from build123d import *

# Parameters (mm, degrees)
SKETCH_W            = 50
SKETCH_H            = 50
PAD_DEPTH           = 4
SKETCH001_W         = 50
SKETCH001_H         = 4
PAD001_DEPTH        = 43
SKETCH002_R         = 11.75
POCKET_DEPTH        = 4.001
HOLE_D              = 4.4
HOLE_CSINK_D        = 8
HOLE_CSINK_ANGLE    = 90
HOLE001_D           = 3.3
HOLE001_DEPTH       = 24.00858
HOLE001_CSINK_D     = 6
HOLE001_CSINK_ANGLE = 90
HOLE001_TIPS_R      = 1.65
SKETCH005_W         = 4
SKETCH005_H         = 46
PAD002_DEPTH        = 43
CHAMFER_SIZE        = 42.99
FILLET_R            = 3.99
FILLET001_R         = 3
POCKET001_DEPTH     = 0.5
POCKET002_DEPTH     = 0.5


with BuildPart() as part:
    # Sketch → Pad (new body)
    with BuildSketch(Plane.XY):
        Rectangle(SKETCH_W, SKETCH_H)
    extrude(amount=PAD_DEPTH)

    # Sketch001 (on Face6 of Pad) → Pad001 (join)
    with BuildSketch(Plane.XY.offset(4)):
        with Locations((0, -23)):
            Rectangle(SKETCH001_W, SKETCH001_H)
    extrude(amount=PAD001_DEPTH)

    # Sketch002 (on Face9 of Pad001) → Pocket (cut, through all)
    with BuildSketch(Plane(origin=(0, -21, 0), x_dir=(-1, 0, 0), z_dir=(0, 1, 0))):
        with Locations((0, 25.5)):
            Circle(SKETCH002_R)
    extrude(amount=-POCKET_DEPTH, mode=Mode.SUBTRACT)

    # Hole (through all)
    with Locations(Plane.XY.offset(4)):
        with Locations((12.5, -7), (-12.5, -7), (-12.5, 18), (12.5, 18)):
            CounterSinkHole(HOLE_D / 2, HOLE_CSINK_D / 2, counter_sink_angle=HOLE_CSINK_ANGLE)

    # Hole001
    with Locations(Plane.XZ.offset(25)):
        with Locations((-15.5, 41), (15.5, 41), (15.5, 10), (-15.5, 10)):
            CounterSinkHole(HOLE001_D / 2, HOLE001_CSINK_D / 2, depth=HOLE001_DEPTH, counter_sink_angle=HOLE001_CSINK_ANGLE)

    # Hole001 tips → Hole001 tip 1 section 0
    with BuildSketch(Plane.XZ.offset(0.99142), mode=Mode.PRIVATE) as hole001_tip_1_s0:
        with Locations((-15.5, 41)):
            Circle(HOLE001_TIPS_R)
    loft([hole001_tip_1_s0.sketch, Vertex(-15.5, 0, 41)], mode=Mode.SUBTRACT)

    # Hole001 tips → Hole001 tip 2 section 0
    with BuildSketch(Plane.XZ.offset(0.99142), mode=Mode.PRIVATE) as hole001_tip_2_s0:
        with Locations((15.5, 41)):
            Circle(HOLE001_TIPS_R)
    loft([hole001_tip_2_s0.sketch, Vertex(15.5, 0, 41)], mode=Mode.SUBTRACT)

    # Hole001 tips → Hole001 tip 3 section 0
    with BuildSketch(Plane.XZ.offset(0.99142), mode=Mode.PRIVATE) as hole001_tip_3_s0:
        with Locations((15.5, 10)):
            Circle(HOLE001_TIPS_R)
    loft([hole001_tip_3_s0.sketch, Vertex(15.5, 0, 10)], mode=Mode.SUBTRACT)

    # Hole001 tips → Hole001 tip 4 section 0
    with BuildSketch(Plane.XZ.offset(0.99142), mode=Mode.PRIVATE) as hole001_tip_4_s0:
        with Locations((-15.5, 10)):
            Circle(HOLE001_TIPS_R)
    loft([hole001_tip_4_s0.sketch, Vertex(-15.5, 0, 10)], mode=Mode.SUBTRACT)

    # Sketch005 (on Face5 of Hole001) → Pad002 (join)
    with BuildSketch(Plane.XY.offset(4)):
        with Locations((23, 2)):
            Rectangle(SKETCH005_W, SKETCH005_H)
        with Locations((-23, 2)):
            Rectangle(SKETCH005_W, SKETCH005_H)
    extrude(amount=PAD002_DEPTH)

    # Chamfer
    chamfer_edges = [part.edges().sort_by_distance(p)[0] for p in [
        (23, 25, 47),
        (-23, 25, 47),
    ]]
    chamfer(chamfer_edges, length=CHAMFER_SIZE)

    # Fillet
    fillet_edges = [part.edges().sort_by_distance(p)[0] for p in [
        (25, -23, 47),
        (-25, -23, 47),
    ]]
    fillet(fillet_edges, radius=FILLET_R)

    # Fillet001
    fillet001_edges = [part.edges().sort_by_distance(p)[0] for p in [
        (25, 25, 2),
        (-25, 25, 2),
    ]]
    fillet(fillet001_edges, radius=FILLET001_R)

    # Fillet001 Face9 → Pocket001 (cut)
    with BuildSketch(Plane(origin=(-21, -5.601727, 19.213451), x_dir=(0, -1, 0), z_dir=(1, 0, 0))):
        Polygon((-30.601727, 15.213451), (-30.601727, 15.203451), (12.388273, -27.786549), (15.398273, -27.786549), (15.398273, 15.213451), align=None)
    extrude(amount=-POCKET001_DEPTH, mode=Mode.SUBTRACT)

    # Pocket001 Face46 → Pocket002 (cut)
    with BuildSketch(Plane(origin=(21, -5.601727, 19.213451), x_dir=(0, 1, 0), z_dir=(-1, 0, 0))):
        Polygon((30.601727, 15.203451), (30.601727, 15.213451), (-15.398273, 15.213451), (-15.398273, -27.786549), (-12.388273, -27.786549), align=None)
    extrude(amount=-POCKET002_DEPTH, mode=Mode.SUBTRACT)


solid = part.part
Could you check a few things on this model? Use its own coordinates, in mm. A direction names the side the tool comes from. Round coordinates to 2 decimals unless told otherwise and drop trailing zeros. Loops run counter-clockwise (first coordinate to the right, second up) from the corner with the lowest first, then second, coordinate; pieces in that order, holes last. Notation, with made-up numbers: (59.25, 88.5) - (95.25, 88.5) arc R31 cw to (95.25, 117.5) - close; hole circle Ø2 at (28.5, -16). An arc over 180 degrees is marked (long way). Write item = value, one per line.
1) Imagine slicing it at A-A (x = 0). Please give me the cut outline in (y, z).
Computed:
outline = (-25, 0) - (25, 0) - (25, 4) - (-21, 4) - (-21, 13.75) - (-25, 13.75) - close; (-25, 37.25) - (-21, 37.25) - (-21, 47) - (-25, 47) - close
2) Imagine slicing it at D-D (y = -1.5). Please give me the cut outline in (x, z).
Computed:
outline = (-25, 0) - (25, 0) - (25, 30.51) - (21.5, 30.51) - (21.5, 4) - (-21.5, 4) - (-21.5, 30.51) - (-25, 30.51) - close
3) Imagine slicing it at C-C (z = 25.5). Please give me the cut outline in (x, y).
Computed:
outline = (-25, -25) - (-11.75, -25) - (-11.75, -21) - (-21.5, -21) - (-21.5, 3.51) - (-25, 3.51) - close; (11.75, -25) - (25, -25) - (25, 3.51) - (21.5, 3.51) - (21.5, -21) - (11.75, -21) - close
4) I need wall thicknesses on line 1 along Y through (x, z) = (-12.5, 1); line 2 along Z through (x, y) = (-15.5, -22.3); line 3 along X through (y, z) = (-22.9, 41). Which ranges of each line are inside material? Lowest first, please. Write a range as from..to.
Computed:
line_1 = -25..-9.2, -4.8..15.8, 20.2..25
line_2 = 0..8.35, 11.65..39.35, 42.65..47
line_3 = -25..-17.15, -13.85..13.85, 17.15..25
5) On a 3-axis mill with a long thin cutter (end or side, diameter ignored), from which of +Z, -Z, +X, -X, +Y, -Y can I reach the whole of each face in a straight line? I mean faces 4 (the flat face through (9, -21, 35)), 5 (the cylindrical face through (13.976, -22.306, 9.368)). Say none if no direction works.
Computed:
face_4 = +Z, +Y
face_5 = +Y, -Y
6) I'm going to push flat-ended pins straight in: P1, Ø3, axis at x = -10.5, z = 6, coming from the +Y side; P2, Ø2.5, axis at x = -15.5, z = 41, coming from the +Y side; P3, Ø4.5, axis at x = 15.5, z = 41, coming from the -Y side; P4, Ø5.5, axis at x = -12.5, y = -7, coming from the +Z side. Where does each tip first touch, or does it pass through?
Computed:
P1 = -21
P2 = through
P3 = -24.25
P4 = 2.75
7) If we mould it in two halves opening along Z, with no side actions, what happens to faces 1 (the cylindrical face through (-16.39, -22.31, 42.39)), 2 (the flat face through (-23.27, 3.82, 25.19)), 3 (the flat face through (21.5, -3, 20))? For each: pulls with the +Z half, pulls with the -Z half, needs draft (parallel to the pull), parting line crosses it, or undercut.
Computed:
face_1 = undercut
face_2 = pulls with the +Z half
face_3 = needs draft
8) Imagine slicing it at B-B (y = -7). Please give me the cut outline in (x, z).
Computed:
outline = (-25, 0) - (-14.7, 0) - (-14.7, 2.2) - (-16.5, 4) - (-21.5, 4) - (-21.5, 36.01) - (-25, 36.01) - close; (-10.3, 0) - (10.3, 0) - (10.3, 2.2) - (8.5, 4) - (-8.5, 4) - (-10.3, 2.2) - close; (14.7, 0) - (25, 0) - (25, 36.01) - (21.5, 36.01) - (21.5, 4) - (16.5, 4) - (14.7, 2.2) - close
